```python
from build123d import *

# Parameters (mm, degrees)
F0_R      = 2.4511
F1_DEPTH  = 6.35
F2_DEPTH  = 3.175
F4_DEPTH  = 22.225
F10_W     = 56.74121622
F10_H     = 63.8059750199
F11_DEPTH = 25.4
F16_W     = 82.6793257147
F16_H     = 72.7323014289
F17_DEPTH = 25.4
F19_DEPTH = 50.8
F20_DEPTH = 25.4


with BuildPart() as f1:
    # F0 (on Right) → F1 (new body)
    with BuildSketch(Plane.YZ):
        Circle(F0_R)
    extrude(amount=F1_DEPTH)

    # F0 (on Right) → F2 (join)
    with BuildSketch(Plane.YZ):
        with BuildLine():
            ThreePointArc((-2.7727080887, -2.2264828441), (1.1801241538, -3.3544661247), (3.556, 0))
            ThreePointArc((3.556, 0), (-1.1801241538, 3.3544661247), (-2.7727080887, -2.2264828441))
        make_face()
        Circle(F0_R, mode=Mode.SUBTRACT)
        with BuildLine():
            ThreePointArc((-2.7727080887, -2.2264828441), (-1.1801241538, 3.3544661247), (3.556, 0))
            Line((3.556, 0), (3.556, 3.81))
            Line((3.556, 3.81), (-9.144, 10.16))
            Line((-9.144, 10.16), (-48.26, 10.16))
            Line((-48.26, 10.16), (-65.4478720941, 15.7807023171))
            ThreePointArc((-65.4478720941, 15.7807023171), (-67.5825080121, 15.0880015075), (-67.5765277328, 12.843793596))
            Line((-67.5765277328, 12.843793596), (-53.34, 3.81))
            Line((-53.34, 3.81), (-8.837933323, 3.81))
            ThreePointArc((-8.837933323, 3.81), (-7.7397247856, 3.5603139541), (-6.8574275453, 2.8603448886))
            Line((-6.8574275453, 2.8603448886), (-2.7727080887, -2.2264828441))
        make_face()
    extrude(amount=F2_DEPTH)

    # F3 (on face) → F4 (join)
    with BuildSketch(Plane.YZ.offset(3.175)):
        with BuildLine():
            Line((-8.837933323, 3.81), (3.556, 3.81))
            Line((3.556, 3.81), (-9.144, 10.16))
            Line((-9.144, 10.16), (-48.26, 10.16))
            Line((-48.26, 10.16), (-65.4478720941, 15.7807023171))
            ThreePointArc((-65.4478720941, 15.7807023171), (-67.5825080121, 15.0880015075), (-67.5765277328, 12.843793596))
            Line((-67.5765277328, 12.843793596), (-53.34, 3.81))
            Line((-53.34, 3.81), (-8.837933323, 3.81))
        make_face()
    extrude(amount=F4_DEPTH)

    # F10 (on 3pt) → F11 (cut)
    with BuildSketch(Plane(origin=(6.888273007, 0, 13.3567620635), x_dir=(0.8887708418, 0, -0.4583518198), z_dir=(0.4583518198, 0, 0.8887708418))):
        with Locations((15.902667772, -15.6232602894)):
            Rectangle(F10_W, F10_H)
    extrude(amount=F11_DEPTH, mode=Mode.SUBTRACT)

    # F16 (on 3pt) → F17 (cut)
    with BuildSketch(Plane(origin=(3.3452742707, 2.6018799884, 6.4229265998), x_dir=(0.9005619877, -0.1632211346, -0.4029230293), z_dir=(-0.4347276232, -0.3381214847, -0.8346770365))):
        with Locations((10.8647113666, 5.6677246466)):
            Rectangle(F16_W, F16_H)
    extrude(amount=-F17_DEPTH, mode=Mode.SUBTRACT)

    # F18 (on face) → F19 (cut)
    with BuildSketch(Plane(origin=(0, -47.5262477994, 0), x_dir=(-1, 0, 0), z_dir=(0, 1, 0))):
        with BuildLine():
            Line((-25.4, 10.16), (-13.0869806094, 10.16))
            ThreePointArc((-13.0869806094, 10.16), (-8.7936537349, 13.9337689195), (-6.7809289321, 19.2838087678))
            Line((-6.7809289321, 19.2838087678), (-25.4, 19.48883757))
            Line((-25.4, 19.48883757), (-25.4, 10.16))
        make_face()
    extrude(amount=-F19_DEPTH, mode=Mode.SUBTRACT)

    # F20 (cut): a face of the model
    f20_faces = [f1.faces().sort_by_distance(p)[0] for p in [
        (21.2956602031, -47.5262477994, 8.0433333333),
    ]]
    extrude(f20_faces, amount=-F20_DEPTH, mode=Mode.SUBTRACT)

    # F21: F1 across plane


with BuildPart() as f1_1:
    add(f1.part)
    add(f1.part.mirror(Plane.YZ))


solid = f1_1.part
```
Here's how the part is built. I have some questions about the finished solid (model axes, mm). A direction names the side the tool comes from. Coordinates: 2 decimals unless noted, no trailing zeros. Order: outer loops, then holes, each group sorted by start corner. A loop starts at its lowest first (then second) coordinate and runs counter-clockwise, first axis right, second up. Notation, with made-up numbers: M 65,37 L 121,37 A23 ccw 121,74 Z; hole C 53.5,79.25 d9. An arc over 180 degrees is marked long. Answer as a JSON object with one key per item and string values. Group by question number.
(1) Suppose I cut it at D-D, the plane y = 0. Please give me the cut outline in (x, z) (3 decimals).
(2) Suppose I cut it at A-A, the plane x = 0. Please give me the cut outline in (y, z), then the cut area to 3 significant figures.
(3) I need wall thicknesses on probe 1 along Z at (x, y) = (9, -42); probe 2 along Z at (x, y) = (3.5, -55); probe 3 along X at (y, z) = (-17.5, 5). Which ranges of each line are inside material? Lowest first, please.
(4) Suppose I cut it at B-B, the plane y = -40. Please give me the cut outline in (x, z), then the cut area to 3 significant figures.
(5) Suppose I cut it at C-C, the plane z = 14. Please give me the cut outline in (x, y).
(6) For pin 1 (4 mm diameter, centred on y = 1, z = 1, fed in from -X); pin 2 (2 mm diameter, centred on y = -10.5, z = 9.5, fed in from +X); pin 3 (10 mm diameter, centred on x = 7.5, y = -17.5, fed in from +Z), each with a flat end and sliding along its axis, tell me the tip position at first contact or that it passes through.
(7) If we mould it in two halves opening along Z, with no side actions, what happens to faces 4 (the face through (-3.175, -3, 1)), 5 (the face through (6.35, 0, 0)), 6 (the face through (19.16, -40.94, 7.03))? For each: released by +Z, released by -Z, zero draft, split by the parting line, or undercut.
(8) Which directions (+Z, -Z, +X, -X, +Y, -Y) give clear straight access to the entire face, cutting with the end or side of a thin tool? Please do faces 1 (the face through (-4.74, 2.338, 0.736)), 2 (the face through (4.74, 2.338, 0.736)), 3 (the face through (0, -28, 10.16)).
Values found:
{
 "1": {"outline": "M -10.386,3.81 L -3.175,3.81 L -3.175,2.451 L -6.35,2.451 L -6.35,-2.451 L -3.175,-2.451 L -3.175,-3.556 L 3.175,-3.556 L 3.175,-2.451 L 6.35,-2.451 L 6.35,2.451 L 3.175,2.451 L 3.175,3.81 L 10.386,3.81 L 6.972,5.588 L -6.972,5.588 Z"},
 "2": {"outline": "M -67.58,12.84 L -53.34,3.81 L -8.84,3.81 A2.54 cw -6.86,2.86 L -2.77,-2.23 A3.56 ccw 3.56,0 L 3.56,3.81 L -9.14,10.16 L -48.26,10.16 L -65.45,15.78 A1.91 ccw Z", "area": "465 mm^2"},
 "3": {"probe 1": "z = 3.81 to 10.16", "probe 2": "z = 4.86 to 12.36", "probe 3": "x = -21.71 to 21.71"},
 "4": {"outline": "M -25.4,3.81 L 25.4,3.81 L 13.09,10.16 L -13.09,10.16 Z", "area": "244 mm^2"},
 "5": {"outline": "M -8.75,-67.94 L 8.75,-67.94 L 8.75,-60 L -8.75,-60 Z"},
 "6": {"pin 1": "stops at x = -6.35", "pin 2": "stops at x = 9.7", "pin 3": "stops at z = 10.16"},
 "7": {"face 4": "undercut", "face 5": "zero draft", "face 6": "released by +Z"},
 "8": {"face 1": "-X", "face 2": "+X", "face 3": "+Z, +X, -X, +Y"}
}
